from build123d import *

# Parameters (mm, degrees)
SKETCH1_W           = 57
SKETCH1_H           = 34
SKETCH1_R           = 5
SKETCH1_R_2         = 1.7
BOSS_EXTRUDE1_DEPTH = 3
SKETCH6_R           = 1.45
BOSS_EXTRUDE3_DEPTH = 2.8


with BuildPart() as part:
    # Sketch1 → Boss-Extrude1 (new body)
    with BuildSketch(Plane(origin=(0, 0, 0), x_dir=(1, 0, 0), z_dir=(0, 1, 0))):
        Rectangle(SKETCH1_W, SKETCH1_H)
        with Locations(Location((0, 0, 0), (0, 0, 270))):
            Circle(SKETCH1_R, mode=Mode.SUBTRACT)
        with Locations(Location((-8.25, 9, 0), (0, 0, 270))):
            Circle(SKETCH1_R_2, mode=Mode.SUBTRACT)
        with Locations(Location((8.25, 9, 0), (0, 0, 270))):
            Circle(SKETCH1_R_2, mode=Mode.SUBTRACT)
        with Locations(Location((8.25, -9, 0), (0, 0, 270))):
            Circle(SKETCH1_R_2, mode=Mode.SUBTRACT)
        with Locations(Location((-8.25, -9, 0), (0, 0, 270))):
            Circle(SKETCH1_R_2, mode=Mode.SUBTRACT)
    extrude(amount=BOSS_EXTRUDE1_DEPTH)

    # Sketch6 → Boss-Extrude3 (add)
    # profile 1 of 4: a face of its own
    with BuildSketch(Plane.XY.offset(17)):
        with BuildLine():
            Line((22.5, 7.238289821), (22.5, 3))
            Line((22.5, 3), (28.5, 3))
            Line((28.5, 3), (28.5, 10.1))
            Line((28.5, 10.1), (24.532387855, 10.1))
            ThreePointArc((24.532387855, 10.1), (23.626017075, 8.591148462), (22.5, 7.238289821))
        make_face()
        with Locations((25.25, 7.25)):
            Circle(SKETCH6_R, mode=Mode.SUBTRACT)
    # profile 2 of 4: a face of its own
    with BuildSketch(Plane.XY.offset(17)):
        with BuildLine():
            Line((0, 10.1), (0, 3))
            Line((0, 3), (6, 3))
            Line((6, 3), (6, 7.238289821))
            ThreePointArc((6, 7.238289821), (4.873982925, 8.591148462), (3.967612145, 10.1))
            Line((3.967612145, 10.1), (0, 10.1))
        make_face()
        with Locations((3.25, 7.25)):
            Circle(SKETCH6_R, mode=Mode.SUBTRACT)
    # profile 3 of 4: a face of its own
    with BuildSketch(Plane.XY.offset(17)):
        with BuildLine():
            Line((-6, 7.238289821), (-6, 3))
            Line((-6, 3), (0, 3))
            Line((0, 3), (0, 10.1))
            Line((0, 10.1), (-3.967612145, 10.1))
            ThreePointArc((-3.967612145, 10.1), (-4.873982925, 8.591148462), (-6, 7.238289821))
        make_face()
        with Locations((-3.25, 7.25)):
            Circle(SKETCH6_R, mode=Mode.SUBTRACT)
    # profile 4 of 4: a face of its own
    with BuildSketch(Plane.XY.offset(17)):
        with BuildLine():
            Line((-28.5, 10.1), (-28.5, 3))
            Line((-28.5, 3), (-22.5, 3))
            Line((-22.5, 3), (-22.5, 7.238289821))
            ThreePointArc((-22.5, 7.238289821), (-23.626017075, 8.591148462), (-24.532387855, 10.1))
            Line((-24.532387855, 10.1), (-28.5, 10.1))
        make_face()
        with Locations((-25.25, 7.25)):
            Circle(SKETCH6_R, mode=Mode.SUBTRACT)
    boss_extrude3 = extrude(amount=-BOSS_EXTRUDE3_DEPTH)

    # Mirror2: Boss-Extrude3 across plane
    add(boss_extrude3.mirror(Plane.XY))


solid = part.part
Could you check a few things on this model? Use its own coordinates, in mm. A direction names the side the tool comes from. Give positions to 0.01 mm unless a question says otherwise; leave off trailing zeros. Order: outer loops, then holes, each group sorted by start corner. A loop starts at its lowest first (then second) coordinate and runs counter-clockwise, first axis right, second up. Notation, with made-up numbers: (33.5, 19) - (86.5, 19) arc R21 cw to (86.5, 35) - close; hole circle Ø10 at (-3, 79). An arc over 180 degrees is marked (long way). One line per item, written item: value. Start each with the question number.
1. If I drill on probe 1 along X at (y, z) = (1.65, 9); probe 2 along Z at (x, y) = (1.5, 9.25); probe 3 along Y at (x, z) = (-3.25, 15.45), over which ranges is the centre line in solid material (lowest first)?
2. Imagine slicing it at C-C on x = 0. List the corners of the cut face in (y, z) for me, plus the area to 3 significant figures.
3. Imagine slicing it at A-A on x = 25.25. List the corners of the cut face in (y, z) for me, plus the area to 3 significant figures.
4. Thinking about a two-plate mould opening in Z: for faces 3 (the face through (-26.2, 5.8, 14.2)), 4 (the face through (0, 3, 17)), 5 (the face through (-26.2, 5.8, -14.2)), 6 (the face through (4.89, 8.57, 15.62)), which applies, +Z half, -Z half, draft (parallel to the pull), parting line (faces both ways), or undercut?
5. Imagine slicing it at D-D on z = 4. List the corners of the cut face in (x, y) for me, plus the area to 3 significant figures.
6. Imagine slicing it at B-B on z = -9. List the corners of the cut face in (x, y) for me, plus the area to 3 significant figures.
7. For faces 1 (the face through (4.89, 8.57, -15.62)), 2 (the face through (26.589, 6.695, 15.62)), which set-ups out of +Z, -Z, +X, -X, +Y, -Y let a thin tool reach every point of the face, with its end or its side?
8. For P1, Ø1, axis at x = -12, z = 2, coming from the -Y side, with a flat end and sliding along its axis, tell me the tip position at first contact or that it passes through.
Values:
1. probe 1: -28.5 to -9.95, -6.55 to 6.55, 9.95 to 28.5
1. probe 2: -17 to -14.2, 14.2 to 17
1. probe 3: 0 to 5.8, 8.7 to 10.1
2. outline: (0, -17) - (10.1, -17) - (10.1, -14.2) - (3, -14.2) - (3, -5) - (0, -5) - close; (0, 5) - (3, 5) - (3, 14.2) - (10.1, 14.2) - (10.1, 17) - (0, 17) - close
2. area: 112 mm²
3. outline: (0, -17) - (5.8, -17) - (5.8, -14.2) - (3, -14.2) - (3, 14.2) - (5.8, 14.2) - (5.8, 17) - (0, 17) - close; (8.7, -17) - (10.1, -17) - (10.1, -14.2) - (8.7, -14.2) - close; (8.7, 14.2) - (10.1, 14.2) - (10.1, 17) - (8.7, 17) - close
3. area: 126 mm²
4. face 3: undercut
4. face 4: +Z half
4. face 5: undercut
4. face 6: draft
5. outline: (-28.5, 0) - (-3, 0) - (-3, 3) - (-28.5, 3) - close; (3, 0) - (28.5, 0) - (28.5, 3) - (3, 3) - close
5. area: 153 mm²
6. outline: (-28.5, 0) - (-9.95, 0) - (-9.95, 3) - (-28.5, 3) - close; (-6.55, 0) - (6.55, 0) - (6.55, 3) - (-6.55, 3) - close; (9.95, 0) - (28.5, 0) - (28.5, 3) - (9.95, 3) - close
6. area: 151 mm²
7. face 1: +Z, -Z, +Y
7. face 2: +Z, -Z
8. P1: y = 0
